Check sheet for the modelled part. Datum: model origin and axes. Units: mm. Face numbers are marked on the shaded views. A direction names the side the tool comes from. Round coordinates to 2 decimals unless told otherwise and drop trailing zeros. Order: outer loops, then holes, each group sorted by start corner. A loop starts at its lowest first (then second) coordinate and runs counter-clockwise, first axis right, second up.
Q1. Set-up check for the marked faces 1, 2 and 3: record each of +Z, -Z, +X, -X, +Y, -Y from which the full face is reachable in a straight line by a thin tool's end or side.
Q2. Scan lines: probe 1 along X at (y, z) = (17.5, 4.35); probe 2 along X at (y, z) = (11.5, 1.1); probe 3 along Y at (x, z) = (3, 1.35). Record each from-to range of solid material in increasing order.
Q3. Mould release check, pull along X, two halves, no side actions. Record for the marked faces 4 and 5: +X half, -X half, draft (parallel to the pull), parting line (faces both ways), or undercut.
Q4. Cross-section at B-B on y = 15.75. Record the cut outline in (x, z).
Q5. Cross-section at D-D on x = 8.5. Record the cut outline in (y, z), then the cut area to 3 significant figures.
Q6. Cross-section at C-C on y = 13.25. Record the cut outline in (x, z), then the cut area to 3 significant figures.
Q7. Cross-section at A-A on z = 0.3. Record the cut outline in (x, y).
Q8. Depth check by flat-ended pin: P1, Ø2, axis at x = 6, z = 2.5, coming from the -Y side; P2, Ø2.5, axis at x = -0.5, z = 2, coming from the +Y side; P3, Ø3, axis at x = 5, z = 3, coming from the -Y side; P4, Ø4, axis at x = 8, y = 23.5, coming from the -Z side. Enter the tip coordinate at first touch or a pass-through.
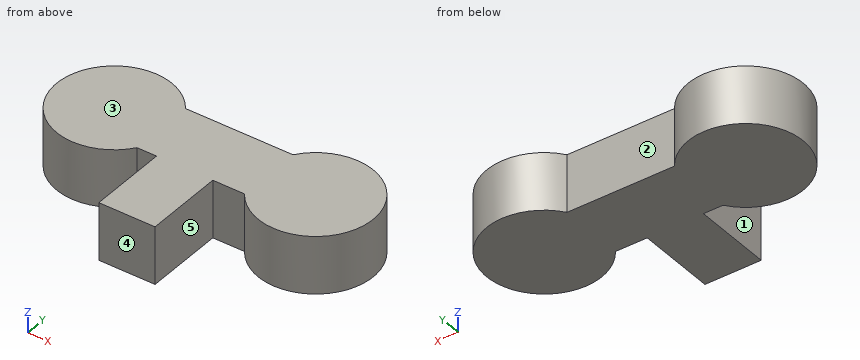
from build123d import *

# Parameters (mm, degrees)
F0_W     = 4.8873469356
F0_H     = 6.8713130732
F1_DEPTH = 5


with BuildPart() as f1:
    # F0 (on Top) → F1 (new body)
    with BuildSketch(Plane.XY):
        Polygon((-3.4519004795, 23.3021316447), (-3.4519004795, 17.5317614882), (-1.7539468208, 17.5317614882), (3.1334001148, 17.5317614882), (5.8841257515, 17.5317614882), (5.8841257515, 23.3021316447), align=None)
        with BuildLine():
            ThreePointArc((-3.4519004795, 23.3021316447), (-12.535490452, 20.4169465664), (-3.4519004795, 17.5317614882))
            Line((-3.4519004795, 17.5317614882), (-3.4519004795, 23.3021316447))
        make_face()
        with Locations((0.689726647, 14.0961049516)):
            Rectangle(F0_W, F0_H)
        with BuildLine():
            ThreePointArc((5.8841257515, 17.5317614882), (14.9677157241, 20.4169465664), (5.8841257515, 23.3021316447))
            Line((5.8841257515, 23.3021316447), (5.8841257515, 17.5317614882))
        make_face()
    extrude(amount=F1_DEPTH)


solid = f1.part
Results found:
1. face 1: +Z, -Z, -Y
1. face 2: +Z, -Z, +Y
1. face 3: +Z, +X, -X, +Y, -Y
2. probe 1: x = -11.6 to -3.47, -1.75 to 3.13, 5.91 to 14.03
2. probe 2: x = -1.75 to 3.13
2. probe 3: y = 10.66 to 23.3
3. face 4: draft
3. face 5: undercut
4. outline: (-9.33, 0) - (-5.74, 0) - (-5.74, 5) - (-9.33, 5) - close; (-1.75, 0) - (3.13, 0) - (3.13, 5) - (-1.75, 5) - close; (8.17, 0) - (11.76, 0) - (11.76, 5) - (8.17, 5) - close
5. outline: (15.64, 0) - (25.2, 0) - (25.2, 5) - (15.64, 5) - close
5. area: 47.8 mm2
6. outline: (-1.75, 0) - (3.13, 0) - (3.13, 5) - (-1.75, 5) - close
6. area: 24.4 mm2
7. outline: (-3.45, 17.53) - (-1.75, 17.53) - (-1.75, 10.66) - (3.13, 10.66) - (3.13, 17.53) - (5.88, 17.53) arc R5 ccw (long way) to (5.88, 23.3) - (-3.45, 23.3) arc R5 ccw (long way) to start
8. P1: stops at y = 16.39
8. P2: stops at y = 23.3
8. P3: stops at y = 16.81
8. P4: stops at z = 0
